from build123d import *

# Parameters (mm, degrees)
M3X0_5_TAPPED_HOLE1_D               = 2.5
M3X0_5_TAPPED_HOLE1_DEPTH           = 5
M3X0_5_TAPPED_HOLE1_TIP             = 0.751075774
M3X0_5_TAPPED_HOLE1_ON_FACE_2_D     = 2.5
M3X0_5_TAPPED_HOLE1_ON_FACE_2_DEPTH = 5
M3X0_5_TAPPED_HOLE1_ON_FACE_2_TIP   = 0.751075774
FILLET1_R                           = 0.1


with BuildPart() as part:
    # Sketch1 → Revolve1 (revolve)
    with BuildSketch(Plane.XY):
        Polygon((0, 0), (20.115, 0), (20.115, 15.7), (10.115, 15.7), (10.115, 16.95), (18.2, 16.95), (18.2, 45.45), (5.5, 45.45), (5.5, 50.85), (0, 50.85), align=None)
    revolve(axis=Axis((0, 50.85, 0), (0, -1, 0)))

    # M3x0.5 Tapped Hole1
    with Locations(Plane(origin=(0, 45.45, -9.5), x_dir=(1, 0, 0), z_dir=(0, 1, 0))):
        with Locations((0, 0), (0, -19)):
            Hole(M3X0_5_TAPPED_HOLE1_D / 2, depth=M3X0_5_TAPPED_HOLE1_DEPTH)
            with Locations((0, 0, -(M3X0_5_TAPPED_HOLE1_DEPTH + M3X0_5_TAPPED_HOLE1_TIP / 2))):  # 118° drill point
                Cone(0, M3X0_5_TAPPED_HOLE1_D / 2, M3X0_5_TAPPED_HOLE1_TIP, mode=Mode.SUBTRACT)

    # M3x0.5 Tapped Hole1 on face 2
    with Locations(Plane(origin=(-16, 0, 0), x_dir=(0, 0, -1), z_dir=(0, -1, 0))):
        with Locations((0, 0), (0, 32)):
            Hole(M3X0_5_TAPPED_HOLE1_ON_FACE_2_D / 2, depth=M3X0_5_TAPPED_HOLE1_ON_FACE_2_DEPTH)
            with Locations((0, 0, -(M3X0_5_TAPPED_HOLE1_ON_FACE_2_DEPTH + M3X0_5_TAPPED_HOLE1_ON_FACE_2_TIP / 2))):  # 118° drill point
                Cone(0, M3X0_5_TAPPED_HOLE1_ON_FACE_2_D / 2, M3X0_5_TAPPED_HOLE1_ON_FACE_2_TIP, mode=Mode.SUBTRACT)

    # Fillet1
    fillet1_edges = [part.edges().sort_by_distance(p)[0] for p in [
        (-18.2, 45.45, 0),
    ]]
    fillet(fillet1_edges, radius=FILLET1_R)


solid = part.part
The model under review builds one solid part; all positions refer to its coordinate system, in mm. A direction names the side the tool comes from. Give positions to 0.01 mm unless a question says otherwise; leave off trailing zeros. Write each loop counter-clockwise with the first axis right and the second up, starting at its lowest first coordinate (ties: lowest second). Pieces come first, ordered by that corner, then holes.
1. Add section A-A, the plane y = 42. Write out the cut boundary in (x, z).
2. Wall thickness on L1, parallel to Z at x = 0, y = 40.5; L2, parallel to Y at x = 11.5, z = 6; L3, parallel to X at y = 41, z = -9: over which ranges is each line inside the solid? List them lowest first.
3. Tool access review of faces 4 (the cylindrical face through (17.054, 2.535, 0.672)), 5 (the flat face through (0, 0, 0)), 6 (the flat face through (-4, 45.45, -4)), 7 (the flat face through (-8, 16.95, -8)): name each direction out of +Z, -Z, +X, -X, +Y, -Y from which nothing blocks a thin tool from reaching the whole face with its end or side.
4. Draft analysis for pull direction Y (two halves, no side actions). For faces 1 (the flat face through (0, 50.85, 0)), 2 (the conical face through (-16.19, 5.62, -0.1)), 3 (the cylindrical face through (-1.32, 16.33, 10.03)), state which applies: +Y half, -Y half, draft (parallel to the pull), parting line (faces both ways), or undercut.
5. For P1, Ø3, axis at y = 10, z = 4, coming from the +X side; P2, Ø12, axis at y = 21.5, z = 5, coming from the +X side; P3, Ø2, axis at x = 16, z = 0, coming from the -Y side, all flat-tipped, find the tip position at first contact; note any pin that passes through.
Worked answers:
1. outline: circle Ø36.4 at (0, 0); hole circle Ø2.5 at (0, -9.5); hole circle Ø2.5 at (0, 9.5)
2. L1: z = -18.2 to -10.75, -8.25 to 8.25, 10.75 to 18.2
2. L2: y = 0 to 15.7, 16.95 to 45.45
2. L3: x = -15.82 to -1.15, 1.15 to 15.82
3. face 4: -Y
3. face 5: +Z, -Z, +X, -X, -Y
3. face 6: +Y
3. face 7: none
4. face 1: +Y half
4. face 2: -Y half
4. face 3: undercut
5. P1: stops at x = 19.96
5. P2: stops at x = 19.81
5. P3: stops at y = 5.15
